The model under review builds one solid part; all positions refer to its coordinate system, in mm. A direction names the side the tool comes from. Coordinates: 2 decimals unless noted, no trailing zeros. Write each loop counter-clockwise with the first axis right and the second up, starting at its lowest first coordinate (ties: lowest second). Pieces come first, ordered by that corner, then holes.
```python
from build123d import *

# Parameters (mm, degrees)
EXTRUDE_1_DEPTH     = 10
SKETCH_3_W          = 20
SKETCH_3_H          = 10
EXTRUDE_2_DEPTH     = 20
FILLET_1_R          = 5
SKETCH_5_R          = 2.15
CUT_EXTRUDE_2_DEPTH = 78.821912081
SKETCH_9_R          = 1
CUT_EXTRUDE_4_DEPTH = 8
SKETCH_10_R         = 5
CUT_EXTRUDE_8_DEPTH = 2


with BuildPart() as part:
    # 스케치2 → 보스-돌출1 (new body)
    with BuildSketch(Plane.XY):
        with BuildLine():
            Line((70, 27.5), (70, 17.5))
            Line((70, 17.5), (50.905124838, 17.5))
            Line((50.905124838, 17.5), (23.200921998, 3.658893602))
            ThreePointArc((23.200921998, 3.658893602), (21.702126319, 2.798642112), (20, 2.5))
            Line((20, 2.5), (-20, 2.5))
            Line((-20, 2.5), (-20, 12.5))
            Line((-20, 12.5), (19.094875162, 12.5))
            Line((19.094875162, 12.5), (46.799078002, 26.341106398))
            ThreePointArc((46.799078002, 26.341106398), (48.297873681, 27.201357888), (50, 27.5))
            Line((50, 27.5), (70, 27.5))
        make_face()
    extrude(amount=EXTRUDE_1_DEPTH)

    # 스케치3 → 보스-돌출2 (add)
    with BuildSketch(Plane.XY.offset(10)):
        with Locations((19.999999999, 7.5)):
            Rectangle(SKETCH_3_W, SKETCH_3_H)
    extrude(amount=-EXTRUDE_2_DEPTH)

    # 필렛1
    fillet_1_edges = [part.edges().sort_by_distance(p)[0] for p in [
        (-20, 12.5, 5),
        (-20, 2.5, 5),
        (70, 17.5, 5),
        (70, 27.5, 5),
    ]]
    fillet(fillet_1_edges, radius=FILLET_1_R - 0.0001)  # a hair under: the kernel refuses the full size

    # 스케치5 → 컷-돌출2 (cut, through all)
    with BuildSketch(Plane(origin=(0, 0, -10), x_dir=(-1, 0, 0), z_dir=(0, 0, -1))):
        with Locations((-19.999999999, 7.5)):
            Circle(SKETCH_5_R)
        with Locations((-65, 22.5)):
            Circle(SKETCH_5_R)
        with Locations((15, 7.5)):
            Circle(SKETCH_5_R)
    extrude(amount=-CUT_EXTRUDE_2_DEPTH, mode=Mode.SUBTRACT)

    # 스케치9 → 컷-돌출4 (cut)
    with BuildSketch(Plane.XZ.offset(-2.5)):
        with Locations(Location((12.499999999, 7.5, 0), (0, 0, 270))):
            Circle(SKETCH_9_R)
        with Locations(Location((27.499999999, 7.5, 0), (0, 0, 270))):
            Circle(SKETCH_9_R)
        with Locations(Location((12.499999999, -7.5, 0), (0, 0, 270))):
            Circle(SKETCH_9_R)
        with Locations(Location((27.499999999, -7.5, 0), (0, 0, 270))):
            Circle(SKETCH_9_R)
    extrude(amount=-CUT_EXTRUDE_4_DEPTH, mode=Mode.SUBTRACT)

    # 스케치10 → 컷-돌출8 (cut)
    with BuildSketch(Plane.XZ.offset(-2.5)):
        with Locations(Location((19.999999999, 0, 0), (0, 0, 270))):
            Circle(SKETCH_10_R)
    extrude(amount=-CUT_EXTRUDE_8_DEPTH, mode=Mode.SUBTRACT)


solid = part.part
```
Item 1: Take a section at B-B, the plane x = 20. Write out the cut boundary in (y, z), plus the area to 3 significant figures.
Solved:
outline: (2.5, -10) - (5.35, -10) - (5.35, 10) - (2.5, 10) - (2.5, 5) - (4.5, 5) - (4.5, -5) - (2.5, -5) - close; (9.65, -10) - (12.5, -10) - (12.5, 0) - (12.95, 0) - (12.95, 10) - (9.65, 10) - close
area: 98.5 mm2
Item 2: Take a section at D-D, the plane x = 6.5. Write out the cut boundary in (y, z), plus the area to 3 significant figures.
Solved:
outline: (2.5, 0) - (12.5, 0) - (12.5, 10) - (2.5, 10) - close
area: 100 mm2
Item 3: Machinability: for faces 1 (the face through (-5, 8, 0)), 2 (the face through (58, 17.5, 5)), 3 (the face through (30, 6, -2)), 4 (the face through (7, 12.5, 2)), 5 (the face through (20, 4.5, 0)), which of the approach directions +Z, -Z, +X, -X, +Y, -Y give a long, thin tool a straight path to every point of the face, cutting with its end or side? Answer none if there is none.
Solved:
face 1: -Z, -X, +Y, -Y
face 2: +Z, -Z, +X, -Y
face 3: -Z, +X, -Y
face 4: -Z, -X, +Y
face 5: -Y
Item 4: For pin 1 (1 mm diameter, centred on x = 27.5, z = 7.5, fed in from -Y); pin 2 (2.5 mm diameter, centred on x = 12.5, z = 7.5, fed in from +Y); pin 3 (2 mm diameter, centred on x = 13, z = 7.5, fed in from -Y); pin 4 (6 mm diameter, centred on x = 27.5, z = 6.5, fed in from +Y), all flat-tipped, find the tip position at first contact; note any pin that passes through.
Solved:
pin 1: stops at y = 10.5
pin 2: stops at y = 12.5
pin 3: stops at y = 2.5
pin 4: stops at y = 18.2
Item 5: Take a section at C-C, the plane z = 7.5. Count the separate pieces of the cut face and the enclosed holes in it, plus the area to 3 significant figures.
Solved:
separate pieces: 1
enclosed holes: 3
area: 851 mm2
Item 6: To check wall thickness, follow line 1 along X through (y, z) = (4.5, -7.5); line 2 along Z through (x, y) = (27.5, 7.5); line 3 along X through (y, z) = (9, 6.25). State the ranges of each line that lie inside material, in increasing order.
Solved:
line 1: x = 10 to 11.5, 13.5 to 26.5, 28.5 to 30
line 2: z = -10 to -8.5, -6.5 to 6.5, 8.5 to 10
line 3: x = -19.77 to -16.54, -13.46 to 18.46, 21.54 to 33.89
Item 7: Take a section at A-A, the plane z = -7.5. Write out the cut boundary in (x, y), plus the area to 3 significant figures.
Solved:
outline: (10, 2.5) - (11.5, 2.5) - (11.5, 10.5) - (13.5, 10.5) - (13.5, 2.5) - (26.5, 2.5) - (26.5, 10.5) - (28.5, 10.5) - (28.5, 2.5) - (30, 2.5) - (30, 12.5) - (10, 12.5) - close; hole circle Ø4.3 at (20, 7.5)
area: 153 mm2
Item 8: Mouldability with a two-part tool opening along Z and no side actions: class faces 6 (the face through (26, 12, 10)), 7 (the face through (28.49, 6.44, 7.63)), 8 (the face through (11.524, 6.444, -7.283)), 9 (the face through (21.585, 8.953, -0.14)) as pulls with the +Z half, pulls with the -Z half, needs draft (parallel to the pull), parting line crosses it, or undercut.
Solved:
face 6: pulls with the +Z half
face 7: undercut
face 8: undercut
face 9: needs draft
